Source: CAD feature listing. Evaluate the final solid. Frame: model axes, mm. Coordinates: 2 decimals unless noted, no trailing zeros. Loops run counter-clockwise (first coordinate to the right, second up) from the corner with the lowest first, then second, coordinate; pieces in that order, holes last.
Item 1: Section query B-B, the plane z = 16. Return the cut outline in (x, y).
Item 2: Line query: probe 1 along Z at (x, y) = (175.5, 0.75); probe 2 along X at (y, z) = (0.9, 42.5); probe 3 along Z at (x, y) = (-7.5, 0.2). Output: solid intervals per line, ascending.
Item 3: Section query A-A, the plane x = 126.5. Return the cut outline in (y, z), then the cut area to 3 significant figures.
Item 4: Section query C-C, the plane y = 0.15. State how many separate pieces and enclosed holes the cut face has, then the cut area to 3 significant figures.
Item 5: Pin query (flat end, axial travel): pin 1 Ø1 at (y, z) = (0.5, 6.5) entering from -X; pin 2 Ø0.6 at (x, y) = (222, 0) entering from -Z. Return the tip coordinate at first contact, or that it passes through.
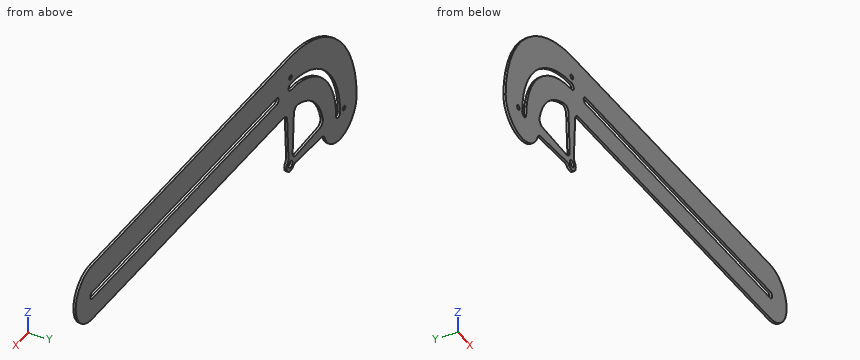
```python
from build123d import *

# Parameters (mm, degrees)
F0_R     = 3
F1_DEPTH = 1
F2_R     = 5
F2_R_2   = 4.99999
F6_DEPTH = 25


# Not quite as in the source:
# - a fillet or chamfer is up to 0.001 mm smaller than in the source, because OpenCascade refuses the exact size
# - a feature of the source that left no trace in its solid (it failed there, or was rolled back) is left out


with BuildPart() as f1:
    # F0 (on Front) → F1 (new body, symmetric)
    with BuildSketch(Plane.XZ):
        with BuildLine():
            ThreePointArc((-70.8333333333, 24.6503324296), (-91.1374306092, 19.0940653956), (-100, 0))
            ThreePointArc((-100, 0), (-77.7052620956, -24.8532001359), (-50.5854754405, -5.3787536225))
            ThreePointArc((-50.5854754405, -5.3787536225), (-50.1467998641, -2.7052620956), (-50, 0))
            ThreePointArc((-50, 0), (-54.1054233512, 13.7264950613), (-65.0733333333, 22.9447442542))
            ThreePointArc((-65.0733333333, 22.9447442542), (-68.0112490695, 11.6391580452), (-69, 0))
            ThreePointArc((-69, 0), (-72, -3), (-75, 0))
            ThreePointArc((-75, 0), (-73.9509972887, 12.5), (-70.8333333333, 24.6503324296))
        make_face()
        with BuildLine():
            ThreePointArc((-50, 0), (-50.1467998641, -2.7052620956), (-50.5854754405, -5.3787536225))
            Line((-50.5854754405, -5.3787536225), (-5.1961524227, -3))
            ThreePointArc((-5.1961524227, -3), (-6, 0), (-5.1961524227, 3))
            Line((-5.1961524227, 3), (-49.7147645476, 5.3331215982))
            ThreePointArc((-49.7147645476, 5.3331215982), (-49.9286402147, 2.6703719425), (-50, 0))
        make_face()
        with BuildLine():
            Line((300, 100), (0, 100))
            ThreePointArc((0, 100), (-70.7106781187, 70.7106781187), (-100, 0))
            ThreePointArc((-100, 0), (-91.1374306092, 19.0940653956), (-70.8333333333, 24.6503324296))
            ThreePointArc((-70.8333333333, 24.6503324296), (-43.4524168935, 61.1300864232), (0, 75))
            ThreePointArc((0, 75), (2.1213203436, 74.1213203436), (3, 72))
            ThreePointArc((3, 72), (2.1213203436, 69.8786796564), (0, 69))
            ThreePointArc((0, 69), (-39.861087833, 56.3213429951), (-65.0733333333, 22.9447442542))
            ThreePointArc((-65.0733333333, 22.9447442542), (-54.1054233512, 13.7264950613), (-50, 0))
            ThreePointArc((-50, 0), (-49.9286402147, 2.6703719425), (-49.7147645476, 5.3331215982))
            ThreePointArc((-49.7147645476, 5.3331215982), (-35.3553390593, 35.3553390593), (-5.3331215982, 49.7147645476))
            ThreePointArc((-5.3331215982, 49.7147645476), (-2.6703719425, 49.9286402147), (0, 50))
            Line((0, 50), (5.3480701549, 50))
            Line((5.3480701549, 50), (300, 50))
            ThreePointArc((300, 50), (284.5889649926, 55.314980315), (275.730677801, 69))
            Line((275.730677801, 69), (21, 69))
            ThreePointArc((21, 69), (18, 72), (21, 75))
            Line((21, 75), (275, 75))
            ThreePointArc((275, 75), (282.3223304703, 92.6776695297), (300, 100))
        make_face()
        with BuildLine():
            Line((3, 5.1961524227), (5.3480701549, 50))
            Line((5.3480701549, 50), (0, 50))
            ThreePointArc((0, 50), (-2.6703719425, 49.9286402147), (-5.3331215982, 49.7147645476))
            Line((-5.3331215982, 49.7147645476), (-3, 5.1961524227))
            ThreePointArc((-3, 5.1961524227), (0, 6), (3, 5.1961524227))
        make_face()
        with BuildLine():
            ThreePointArc((-5.1961524227, 3), (-6, 0), (-5.1961524227, -3))
            ThreePointArc((-5.1961524227, -3), (1.5529142706, -5.7955549577), (6, 0))
            ThreePointArc((6, 0), (5.1961524227, 3), (3, 5.1961524227))
            ThreePointArc((3, 5.1961524227), (0, 6), (-3, 5.1961524227))
            ThreePointArc((-3, 5.1961524227), (-4.2426406871, 4.2426406871), (-5.1961524227, 3))
        make_face()
        Circle(F0_R, mode=Mode.SUBTRACT)
        with BuildLine():
            ThreePointArc((325, 75), (317.6776695297, 92.6776695297), (300, 100))
            ThreePointArc((300, 100), (282.3223304703, 92.6776695297), (275, 75))
            Line((275, 75), (300, 75))
            ThreePointArc((300, 75), (302.1213203436, 74.1213203436), (303, 72))
            ThreePointArc((303, 72), (302.1213203436, 69.8786796564), (300, 69))
            Line((300, 69), (275.730677801, 69))
            ThreePointArc((275.730677801, 69), (284.5889649926, 55.314980315), (300, 50))
            ThreePointArc((300, 50), (317.6776695297, 57.3223304703), (325, 75))
        make_face()
    extrude(amount=F1_DEPTH, both=True)

    # F2 (call 1 of 8: OpenCascade refuses the feature's edges together)
    f2_edges = [f1.edges().sort_by_distance(p)[0] for p in [
        (-49.714765, 0, 5.333122),
    ]]
    fillet(f2_edges, radius=F2_R)

    # F2#2 (call 2 of 8)
    f2_2_edges = [f1.edges().sort_by_distance(p)[0] for p in [
        (5.34807, 0, 50),
    ]]
    fillet(f2_2_edges, radius=F2_R)

    # F2#3 (call 3 of 8)
    f2_3_edges = [f1.edges().sort_by_distance(p)[0] for p in [
        (-5.333122, 0, 49.714765),
    ]]
    fillet(f2_3_edges, radius=F2_R)

    # F2#4 (call 4 of 8)
    f2_4_edges = [f1.edges().sort_by_distance(p)[0] for p in [
        (-5.196152, 0, -3),
    ]]
    fillet(f2_4_edges, radius=F2_R)

    # F2#5 (call 5 of 8)
    f2_5_edges = [f1.edges().sort_by_distance(p)[0] for p in [
        (-50.585475, 0, -5.378754),
    ]]
    fillet(f2_5_edges, radius=F2_R)

    # F2#6 (call 6 of 8)
    f2_6_edges = [f1.edges().sort_by_distance(p)[0] for p in [
        (-5.196152, 0, 3),
    ]]
    fillet(f2_6_edges, radius=F2_R)

    # F2#7 (call 7 of 8) (radius 5 in the source; OpenCascade refuses exactly that, so slightly less here)
    f2_7_edges = [f1.edges().sort_by_distance(p)[0] for p in [
        (-3, 0, 5.196152),
    ]]
    fillet(f2_7_edges, radius=F2_R_2)

    # F2#8 (call 8 of 8)
    f2_8_edges = [f1.edges().sort_by_distance(p)[0] for p in [
        (3, 0, 5.196152),
    ]]
    fillet(f2_8_edges, radius=F2_R)

    # F5 (on face) → F6 (cut)
    with BuildSketch(Plane.XZ.offset(1)):
        with BuildLine():
            Line((-82, 0), (-79, 0))
            ThreePointArc((-79, 0), (-80.6813707911, 1.9744557294), (-82.8984754272, 0.629119267))
            Line((-82.8984754272, 0.629119267), (-82, 0))
        make_face()
        with BuildLine():
            ThreePointArc((-82.8984754272, -0.629119267), (-80.6813707911, -1.9744557294), (-79, 0))
            Line((-79, 0), (-82, 0))
            Line((-82, 0), (-82.8984754272, -0.629119267))
        make_face()
        with BuildLine():
            ThreePointArc((-0.629119267, 82.8984754272), (-1.9744557294, 80.6813707911), (0, 79))
            Line((0, 79), (0, 82))
            Line((0, 82), (-0.629119267, 82.8984754272))
        make_face()
        with BuildLine():
            Line((0, 82), (0, 79))
            ThreePointArc((0, 79), (1.4142135624, 79.5857864376), (2, 81))
            ThreePointArc((2, 81), (1.6214559097, 82.1708461611), (0.629119267, 82.8984754272))
            Line((0.629119267, 82.8984754272), (0, 82))
        make_face()
    extrude(amount=-F6_DEPTH, mode=Mode.SUBTRACT)


solid = f1.part
```
Verdict:
1. outline: (-98.71, -1) - (-73.27, -1) - (-73.27, 1) - (-98.71, 1) - close; (-67.12, -1) - (-47.37, -1) - (-47.37, 1) - (-67.12, 1) - close; (-3.57, -1) - (3.57, -1) - (3.57, 1) - (-3.57, 1) - close
2. probe 1: z = 50 to 69, 75 to 100
2. probe 2: x = -90.52 to -61.8, -54.36 to -26.34, -4.96 to 4.96
2. probe 3: z = -3.12 to 3.21, 48.18 to 68.59, 74.62 to 99.72
3. outline: (-1, 50) - (1, 50) - (1, 69) - (-1, 69) - close; (-1, 75) - (1, 75) - (1, 100) - (-1, 100) - close
3. area: 88.0 mm2
4. separate pieces: 1
4. enclosed holes: 6
4. area: 21,300 mm2
5. pin 1: stops at x = -99.82
5. pin 2: stops at z = 50
